Work out the finished part from the listing and answer in its coordinate system (mm). A direction names the side the tool comes from. Give positions to 0.01 mm unless a question says otherwise; leave off trailing zeros. Loops run counter-clockwise (first coordinate to the right, second up) from the corner with the lowest first, then second, coordinate; pieces in that order, holes last.
from build123d import *

# Parameters (mm, degrees)
SKETCH_1_R   = 1.1
SKETCH_1_R_2 = 1.240624
PAD_DEPTH    = 3


with BuildPart() as part:
    # Sketch_1 → Pad (new body)
    with BuildSketch(Plane.XY):
        with BuildLine():
            ThreePointArc((1.767767, 1.767767), (-1.767767, 1.767767), (-1.767767, -1.767767))
            Line((-1.767767, -1.767767), (4.836212, -8.371746))
            Line((4.836212, -8.371746), (4.836212, -78.366013))
            Line((4.836212, -78.366013), (-14.796054, -102.373325))
            ThreePointArc((-14.796054, -102.373325), (-14.44337, -105.891224), (-10.925471, -105.53854))
            Line((9.09799, -81.052855), (-10.925471, -105.53854))
            Line((9.09799, -5.562456), (9.09799, -81.052855))
            Line((1.767767, 1.767767), (9.09799, -5.562456))
        make_face()
        with Locations((-12.860762, -103.955933)):
            Circle(SKETCH_1_R, mode=Mode.SUBTRACT)
        Circle(SKETCH_1_R, mode=Mode.SUBTRACT)
        with Locations((4.297746, -4.297745)):
            Circle(SKETCH_1_R_2, mode=Mode.SUBTRACT)
    extrude(amount=PAD_DEPTH)


solid = part.part
Item 1: Find section D-D, the plane y = -15. Write down the section's boundary in (x, z), plus the area to 3 significant figures.
Item 2: Find section A-A, the plane x = 0. Write down the section's boundary in (y, z), plus the area to 3 significant figures.
Item 3: Consider line 1 (Y direction, x = 0, z = 1.05); line 2 (X direction, y = -46, z = 0.65); line 3 (Y direction, x = -12.75, z = 0.7). Determine where each line is inside the solid, lowest interval first.
Item 4: Determine the mould class of faces 1 (the face through (1.05, 0.33, 1.48)), 2 (the face through (5, -52, 3)), 3 (the face through (-4.84, -90.2, 1.48)) for opening direction X: released by +X, released by -X, zero draft, split by the parting line, or undercut.
Item 5: Flat-ended cylindrical pins translate along their axes: pin 1 Ø1.5 at (y, z) = (-38.5, 2) entering from -X; pin 2 Ø1.8 at (x, y) = (0, 0) entering from +Z. Find the tip coordinate at first contact, or state that the pin passes through.
Item 6: For faces 4 (the face through (9.098, -43, 1)), 5 (the face through (1.488, -5.024, 1.479)), determine the directions among +Z, -Z, +X, -X, +Y, -Y from which every point of the face is accessible in a straight line to the end or side of a thin tool.
Item 7: Find section B-B, the plane y = 0. Write down the section's boundary in (x, z), plus the area to 3 significant figures.
Item 8: Find section C-C, the plane z = 0.5. Write down the section's boundary in (x, y).
Ans:
1. outline: (4.84, 0) - (9.1, 0) - (9.1, 3) - (4.84, 3) - close
1. area: 12.8 mm2
2. outline: (-92.18, 0) - (-84.28, 0) - (-84.28, 3) - (-92.18, 3) - close; (-3.54, 0) - (-1.1, 0) - (-1.1, 3) - (-3.54, 3) - close; (1.1, 0) - (2.5, 0) - (2.5, 3) - (1.1, 3) - close
2. area: 35.2 mm2
3. line 1: y = -92.18 to -84.28, -3.54 to -1.1, 1.1 to 2.5
3. line 2: x = 4.84 to 9.1
3. line 3: y = -106.45 to -105.05, -102.86 to -99.87
4. face 1: undercut
4. face 2: zero draft
4. face 3: released by -X
5. pin 1: stops at x = 4.84
5. pin 2: passes through
6. face 4: +Z, -Z, +X, +Y, -Y
6. face 5: +Z, -Z, -X
7. outline: (-2.5, 0) - (-1.1, 0) - (-1.1, 3) - (-2.5, 3) - close; (1.1, 0) - (3.54, 0) - (3.54, 3) - (1.1, 3) - close
7. area: 11.5 mm2
8. outline: (-14.8, -102.37) arc R2.5 ccw to (-10.93, -105.54) - (9.1, -81.05) - (9.1, -5.56) - (1.77, 1.77) arc R2.5 ccw to (-1.77, -1.77) - (4.84, -8.37) - (4.84, -78.37) - close; hole circle Ø2.2 at (-12.86, -103.96); hole circle Ø2.2 at (0, 0); hole circle Ø2.48 at (4.3, -4.3)
